```python
from build123d import *

# Parameters (mm, degrees)
BOSS_EXTRUDE1_DEPTH = 9.75
CUT_EXTRUDE3_START  = -4.875
CUT_EXTRUDE3_DEPTH  = 4.875
SKETCH3_R           = 2.825
CUT_EXTRUDE4_DEPTH  = 3


with BuildPart() as part:
    # Sketch1 → Boss-Extrude1 (new body)
    with BuildSketch(Plane(origin=(0, 0, 0), x_dir=(1, 0, 0), z_dir=(0, 1, 0))):
        with BuildLine():
            Line((0, 5), (0, 0))
            Line((0, 0), (53.75, 0))
            ThreePointArc((53.75, 0), (55.214466094, 3.535533906), (58.75, 5))
            Line((58.75, 5), (0, 5))
        make_face()
        with BuildLine():
            Line((53.75, 0), (0, 0))
            Line((0, 0), (0, -5.049027621))
            Line((0, -5.049027621), (58.75, -5.049027621))
            Line((58.75, -5.049027621), (58.75, -5))
            ThreePointArc((58.75, -5), (55.214466094, -3.535533906), (53.75, 0))
        make_face()
        with BuildLine():
            ThreePointArc((63.75, 0), (62.285533906, 3.535533906), (58.75, 5))
            Line((58.75, 5), (58.75, 1.5))
            ThreePointArc((58.75, 1.5), (59.810660172, 1.060660172), (60.25, 0))
            ThreePointArc((60.25, 0), (59.810660172, -1.060660172), (58.75, -1.5))
            Line((58.75, -1.5), (58.75, -5))
            ThreePointArc((58.75, -5), (62.285533906, -3.535533906), (63.75, 0))
        make_face()
        with BuildLine():
            ThreePointArc((58.75, 5), (55.214466094, 3.535533906), (53.75, 0))
            Line((53.75, 0), (57.25, 0))
            ThreePointArc((57.25, 0), (57.689339828, 1.060660172), (58.75, 1.5))
            Line((58.75, 1.5), (58.75, 5))
        make_face()
        with BuildLine():
            Line((57.25, 0), (53.75, 0))
            ThreePointArc((53.75, 0), (55.214466094, -3.535533906), (58.75, -5))
            Line((58.75, -5), (58.75, -1.5))
            ThreePointArc((58.75, -1.5), (57.689339828, -1.060660172), (57.25, 0))
        make_face()
    boss_extrude1 = extrude(amount=BOSS_EXTRUDE1_DEPTH)

    # Mirror1: Boss-Extrude1 across plane
    add(boss_extrude1.mirror(Plane(origin=(0, 0, 0), x_dir=(0, 0, 1), z_dir=(1, 0, 0))))

    # Sketch2 → Cut-Extrude3 (cut)
    with BuildSketch(Plane(origin=(0, 9.75, 0), x_dir=(1, 0, 0), z_dir=(0, 1, 0)).offset(CUT_EXTRUDE3_START)):
        with BuildLine():
            Line((60.25, 0), (63.75, 0))
            ThreePointArc((63.75, 0), (62.285533906, 3.535533906), (58.75, 5))
            Line((58.75, 5), (53.75, 5))
            Line((53.75, 5), (53.75, 0))
            Line((53.75, 0), (57.25, 0))
            ThreePointArc((57.25, 0), (58.75, 1.5), (60.25, 0))
        make_face()
        with BuildLine():
            ThreePointArc((58.75, -5), (62.285533906, -3.535533906), (63.75, 0))
            Line((63.75, 0), (60.25, 0))
            ThreePointArc((60.25, 0), (58.75, -1.5), (57.25, 0))
            Line((57.25, 0), (53.75, 0))
            Line((53.75, 0), (53.75, -5.049027621))
            Line((53.75, -5.049027621), (58.75, -5.049027621))
            Line((58.75, -5.049027621), (58.75, -5))
        make_face()
    cut_extrude3 = extrude(amount=CUT_EXTRUDE3_DEPTH, mode=Mode.SUBTRACT)

    # Mirror2: Cut-Extrude3 across plane
    add(cut_extrude3.mirror(Plane(origin=(0, 0, 0), x_dir=(0, 0, 1), z_dir=(1, 0, 0))), mode=Mode.SUBTRACT)

    # Sketch3 → Cut-Extrude4 (cut)
    with BuildSketch(Plane(origin=(0, 0, 0), x_dir=(-1, 0, 0), z_dir=(0, -1, 0))):
        with Locations(Location((58.75, 0, 0), (0, 0, 90))):
            Circle(SKETCH3_R)
        with Locations(Location((-58.75, 0, 0), (0, 0, 90))):
            Circle(SKETCH3_R)
    extrude(amount=-CUT_EXTRUDE4_DEPTH, mode=Mode.SUBTRACT)


solid = part.part
```
Read the model definition and answer for the solid it produces. Units are mm, in the model's axes. A direction names the side the tool comes from. Give positions to 0.01 mm unless a question says otherwise; leave off trailing zeros. Write item = value, one per line. Start each with the question number.
Item 1: A tool of negligible diameter and unlimited length cuts with its end or side. For faces 1 (the flat face through (57.5, 3, -1.2)), 2 (the flat face through (1, 5, 5.049)), 3 (the flat face through (-57.6, 4.875, -1.2)), 4 (the flat face through (53.75, 7, 0)), from which of +Z, -Z, +X, -X, +Y, -Y can it reach the whole face along a straight path? Write none if from no direction.
Item 2: Each of these flat-tipped pins is pushed along its axis until it touches: P1, Ø2.5, axis at y = 7.5, z = 2, coming from the +X side; P2, Ø3, axis at x = -1, z = -3, coming from the -Y side; P3, Ø1.7, axis at x = 57.5, z = 0, coming from the -Y side; P4, Ø2.5, axis at y = 6.5, z = -1, coming from the -X side. Where does it stop, or does it pass through?
Item 3: The mould has two halves that part along X. Classify faces 5 (the flat face through (1, 9.75, 0)), 6 (the cylindrical face through (55.99, 1.48, 0.61)), 7 (the flat face through (-53.75, 7, 0)): +X half, -X half, draft (parallel to the pull), parting line (faces both ways), or undercut.
Item 4: Find the intervals of material crossed by probe 1 along X at (y, z) = (3.75, -0.25); probe 2 along X at (y, z) = (1.7, 0) (3 decimals); probe 3 along X at (y, z) = (7, -0.25), in increasing order. Write a range as [from, to].
Response:
q1.face_1 = -Y
q1.face_2 = +Z, +X, -X, +Y, -Y
q1.face_3 = +Z, -Z, -X, +Y
q1.face_4 = +Z, -Z, +X, +Y
q2.P1 = 53.75
q2.P2 = 0
q2.P3 = 3
q2.P4 = -53.75
q3.face_5 = draft
q3.face_6 = undercut
q3.face_7 = -X half
q4.probe_1 = [-63.74, -60.23], [-57.27, 57.27], [60.23, 63.74]
q4.probe_2 = [-63.75, -61.575], [-55.925, 55.925], [61.575, 63.75]
q4.probe_3 = [-53.75, 53.75]
